For this review, take the finished solid that the model builds, in its own axes (mm). Coordinates: 2 decimals unless noted, no trailing zeros. Write each loop counter-clockwise with the first axis right and the second up, starting at its lowest first coordinate (ties: lowest second). Pieces come first, ordered by that corner, then holes.
Autodesk Inventor part; units mm, degrees
ref_plane "YZ Plane" through (0, 0, 0) normal (1, 0, 0) x (0, 1, 0)
ref_plane "XZ Plane" through (0, 0, 0) normal (0, 1, 0) x (-1, 0, 0)
ref_plane "XY Plane" through (0, 0, 0) normal (0, 0, 1) x (1, 0, 0)
ref_plane "Plano de trabajo1" through (0, 0, 0) normal (0, 0, 1) x (1, 0, 0)
sketch "Boceto1" plane through (0, 0, 0) normal (0, 0, 1) x (1, 0, 0)
  arc A0 (23.25, 32) -> (26.25, 35) centre (23.25, 35) ccw
  line L0 (23.25, 32) -> (10.75, 32)
  arc A1 (7.75, 35) -> (10.75, 32) centre (10.75, 35) ccw
  line L1 (7.75, 35) -> (7.75, 57)
  arc A2 (26.25, 57) -> (7.75, 57) centre (17, 57) ccw
  line L2 (26.25, 57) -> (26.25, 35)
  circle A3 centre (12.75, 37) radius 2.5
  circle A4 centre (21.25, 37) radius 2.5
  circle A5 centre (17, 57) radius 8.5
  arc A6 (15.882, 58) -> (18.118, 58) centre (17, 57) ccw
  circle A7 centre (17, 57) radius 1.75
  circle A8 centre (12.75, 37) radius 1.5
  circle A9 centre (21.25, 37) radius 1.5
  point P0 (0, 0)
  dimension "d0" = 3.5
  dimension "d1" = 3
  dimension "d2" = 3
extrude "Extrusión1" add sketch "Boceto1" along normal blind 2 contours L0 A1 L1 A2 L2 A0 | A3 | A4 | A5
sketch "Boceto2" plane through (0, 0, 0) normal (0, 0, -1) x (-1, 0, 0)
  circle A0 centre (-17, 57) radius 1.75
  circle A1 centre (-17, 57) radius 2.5
  point P0 (0, 0)
  dimension "d5" = 5
extrude "Extrusión2" add sketch "Boceto2" along normal blind 2
fillet "Empalme1" radius 2 1 edges at (19.5, 57, 0)
properties part number "Soporte Motor2"
Q1. Add section C-C (x = 11.75). State the section outline as (y, z) points, then the cut area to 3 significant figures.
Ans:
outline: (32, 0) - (35.88, 0) - (35.88, 2) - (32, 2) - close; (38.12, 0) - (64.62, 0) - (64.62, 2) - (38.12, 2) - close
area: 60.8 mm2
Q2. Add section D-D (z = -1.6). State the section outline as (x, y) points.
Ans:
outline: circle Ø5.08 at (17, 57); hole circle Ø3.5 at (17, 57)
Q3. For probe 1 along Y at (x, z) = (17, 1.45); probe 2 along X at (y, z) = (57, 1.4); probe 3 along X at (y, z) = (57, -1.4), list the stretches that pass through material, from the lowest coordinate up.
Ans:
probe 1: y = 32 to 55.25, 58.75 to 66.25
probe 2: x = 7.75 to 15.25, 18.75 to 26.25
probe 3: x = 14.41 to 15.25, 18.75 to 19.59
Q4. Add section B-B (y = 37). State the section outline as (x, z) points, then the cut area to 3 significant figures.
Ans:
outline: (7.75, 0) - (11.25, 0) - (11.25, 2) - (7.75, 2) - close; (14.25, 0) - (19.75, 0) - (19.75, 2) - (14.25, 2) - close; (22.75, 0) - (26.25, 0) - (26.25, 2) - (22.75, 2) - close
area: 25.0 mm2
Q5. Draft analysis for pull direction X (two halves, no side actions). For faces 1 (the cylindrical face through (20.06, 37.91, 0.99)), 2 (the flat face through (16, 59, -2)), 3 (the cylindrical face through (25.39, 32.9, 0.99)), state which applies: +X half, -X half, draft (parallel to the pull), parting line (faces both ways), or undercut.
Ans:
face 1: undercut
face 2: draft
face 3: +X half
